Answer from the drawing. Dimensions are ordinates in mm from the lowest x, y and z of the part. Give positions to 0.01 mm unless a question says otherwise; leave off trailing zeros. Loops run counter-clockwise (first coordinate to the right, second up) from the corner with the lowest first, then second, coordinate; pieces in that order, holes last. Notation, with made-up numbers: (32, -31.5) -> (59, -31.5) arc R9 ccw to (59, -24.5) -> close; hole circle Ø1 at (47.5, 17). An arc over 180 degrees is marked (long way). Answer as CSV lines item,"result". Start each with the question number.
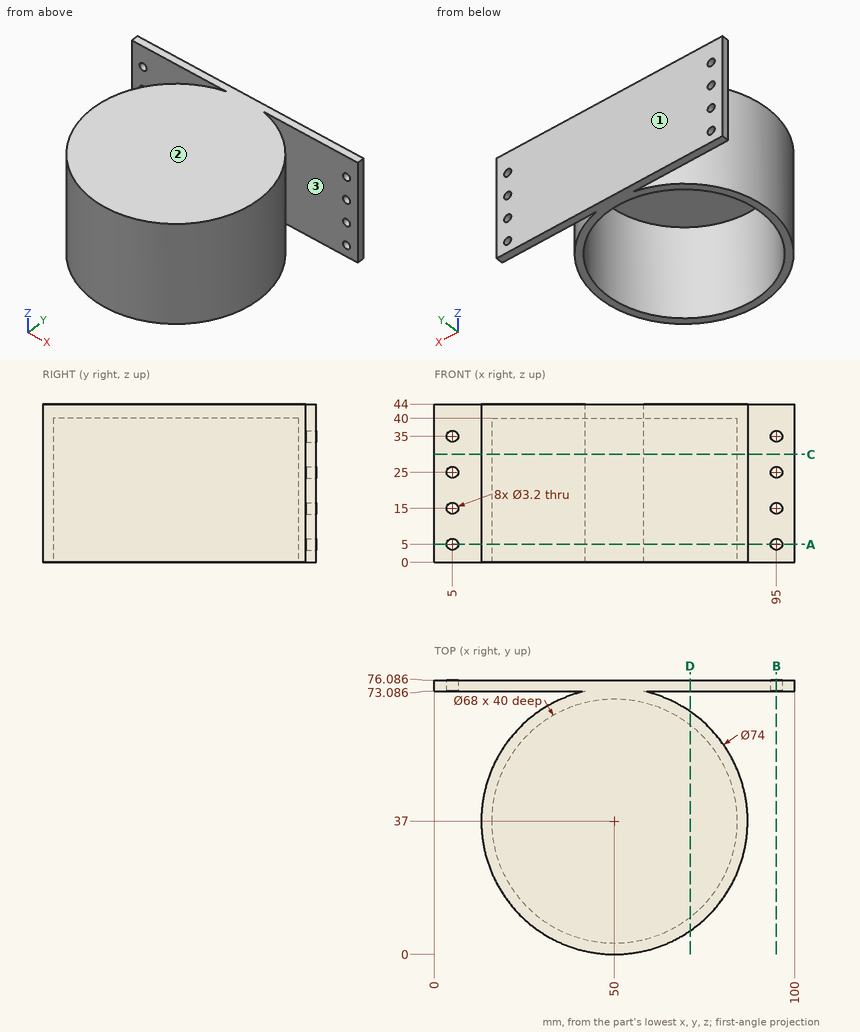
(1) Find section C-C on z = 30. Write down the section's boundary in (x, y), then the cut area to 3 significant figures.
(2) The mould has two halves that part along Y. Classify the marked faces 1, 2 and 3: pulls with the +Y half, pulls with the -Y half, needs draft (parallel to the pull), parting line crosses it, or undercut.
(3) Find section A-A on z = 5. Write down the section's boundary in (x, y).
(4) Find the intervals of material crossed by line 1 along X through (y, z) = (75, 15); line 2 along Z through (x, y) = (95, 74.5); line 3 along Y through (x, z) = (78.5, 38) (1 decimal), in increasing order. Write a range as from..to.
(5) Find section D-D on x = 71. Write down the section's boundary in (y, z).
(6) Find section B-B on x = 95. Write down the section's boundary in (y, z).
(7) Each of these flat-tipped pins is pushed along its axis until it touches: P1, Ø10, axis at x = 25, z = 4.5, coming from the -Y side; P2, Ø8, axis at x = 48.5, y = 11.5, coming from the -Z side; P3, Ø6, axis at y = 12, z = 15.5, coming from the +X side. Where does it stop, or does it pass through?
Answer block:
1,outline,"(0, 73.09) -> (41.83, 73.09) arc R37 ccw (long way) to (58.17, 73.09) -> (100, 73.09) -> (100, 76.09) -> (0, 76.09) -> close; hole circle Ø68 at (50, 37)"
1,area,"959 mm2"
2,face 1,"pulls with the +Y half"
2,face 2,"needs draft"
2,face 3,"undercut"
3,outline,"(0, 73.09) -> (3.4, 73.09) -> (3.4, 76.09) -> (0, 76.09) -> close; (6.6, 73.09) -> (41.83, 73.09) arc R37 ccw (long way) to (58.17, 73.09) -> (93.4, 73.09) -> (93.4, 76.09) -> (6.6, 76.09) -> close; (96.6, 73.09) -> (100, 73.09) -> (100, 76.09) -> (96.6, 76.09) -> close; hole circle Ø68 at (50, 37)"
4,line 1,"x = 0..3.4, 6.6..93.4, 96.6..100"
4,line 2,"z = 0..3.4, 6.6..13.4, 16.6..23.4, 26.6..33.4, 36.6..44"
4,line 3,"y = 13.4..18.5, 55.5..60.6, 73.1..76.1"
5,outline,"(6.54, 0) -> (10.26, 0) -> (10.26, 40) -> (63.74, 40) -> (63.74, 0) -> (67.46, 0) -> (67.46, 44) -> (6.54, 44) -> close; (73.09, 0) -> (76.09, 0) -> (76.09, 44) -> (73.09, 44) -> close"
6,outline,"(73.09, 0) -> (76.09, 0) -> (76.09, 3.4) -> (73.09, 3.4) -> close; (73.09, 6.6) -> (76.09, 6.6) -> (76.09, 13.4) -> (73.09, 13.4) -> close; (73.09, 16.6) -> (76.09, 16.6) -> (76.09, 23.4) -> (73.09, 23.4) -> close; (73.09, 26.6) -> (76.09, 26.6) -> (76.09, 33.4) -> (73.09, 33.4) -> close; (73.09, 36.6) -> (76.09, 36.6) -> (76.09, 44) -> (73.09, 44) -> close"
7,P1,"stops at y = 5.87"
7,P2,"stops at z = 40"
7,P3,"stops at x = 79.75"
